```python
from build123d import *

# Parameters (mm, degrees)
ESBO_O1_R                = 10
RESSALTO_EXTRUS_O1_DEPTH = 6
RESSALTO_EXTRUS_O2_START = -4.5
RESSALTO_EXTRUS_O2_DEPTH = 4.5
FILETE1_R                = 3
FILETE2_R                = 1
FILETE3_R                = 10
ESBO_O3_R                = 4
RESSALTO_EXTRUS_O3_DEPTH = 10
ESBO_O4_R                = 3.3
CORTE_EXTRUS_O1_DEPTH    = 14


with BuildPart() as part:
    # Esboço1 → Ressalto-extrusão1 (new body)
    with BuildSketch(Plane.XY):
        Circle(ESBO_O1_R)
    extrude(amount=RESSALTO_EXTRUS_O1_DEPTH)

    # Esboço2 → Ressalto-extrusão2 (add)
    with BuildSketch(Plane.XY.offset(6).offset(RESSALTO_EXTRUS_O2_START)):
        with BuildLine():
            Line((-9.797958971, 2), (-37.5, 2))
            Line((-37.5, 2), (-37.5, -5))
            ThreePointArc((-37.5, -5), (-36, -6.5), (-34.5, -5))
            Line((-34.5, -5), (-34.5, -2))
            Line((-34.5, -2), (-9.797958971, -2))
            ThreePointArc((-9.797958971, -2), (-10, 0), (-9.797958971, 2))
        make_face()
    extrude(amount=RESSALTO_EXTRUS_O2_DEPTH)

    # Filete1
    filete1_edges = [part.edges().sort_by_distance(p)[0] for p in [
        (-37.5, 2, 3.75),
    ]]
    fillet(filete1_edges, radius=FILETE1_R)

    # Filete2
    filete2_edges = [part.edges().sort_by_distance(p)[0] for p in [
        (-34.5, -2, 3.75),
    ]]
    fillet(filete2_edges, radius=FILETE2_R)

    # Filete3
    filete3_edges = [part.edges().sort_by_distance(p)[0] for p in [
        (-9.797958971, 2, 3.75),
        (-9.797958971, -2, 3.75),
    ]]
    fillet(filete3_edges, radius=FILETE3_R)

    # Esboço3 → Ressalto-extrusão3 (add)
    with BuildSketch(Plane.XY.offset(6)):
        Circle(ESBO_O3_R)
    extrude(amount=RESSALTO_EXTRUS_O3_DEPTH)

    # Esboço4 → Corte-extrusão1 (cut)
    with BuildSketch(Plane.XY.offset(16)):
        Circle(ESBO_O4_R)
    extrude(amount=-CORTE_EXTRUS_O1_DEPTH, mode=Mode.SUBTRACT)


solid = part.part
```
Here's how the part is built. I have some questions about the finished solid (model axes, mm). A direction names the side the tool comes from. Coordinates: 2 decimals unless noted, no trailing zeros. Order: outer loops, then holes, each group sorted by start corner. A loop starts at its lowest first (then second) coordinate and runs counter-clockwise, first axis right, second up. Notation, with made-up numbers: (80, -5.75) -> (106, -5.75) arc R33 cw to (106, 27.25) -> close; hole circle Ø10 at (-23, 24). An arc over 180 degrees is marked (long way). Return JSON: item names as keys, results as strings.
1) If we section it at B-B on x = 0: List the corners of the cut face in (y, z) for me, plus the area to 3 significant figures.
Conclusion:
{"outline": "(-10, 0) -> (10, 0) -> (10, 6) -> (4, 6) -> (4, 16) -> (3.3, 16) -> (3.3, 2) -> (-3.3, 2) -> (-3.3, 16) -> (-4, 16) -> (-4, 6) -> (-10, 6) -> close", "area": "108 mm²"}
2) If we section it at A-A on z = 4.75: List the corners of the cut face in (x, y) for me.
Conclusion:
{"outline": "(-37.5, -5) arc R1.5 ccw to (-34.5, -5) -> (-34.5, -3) arc R1 cw to (-33.5, -2) -> (-16, -2) arc R10 cw to (-8, -6) arc R10 ccw (long way) to (-8, 6) arc R10 cw to (-16, 2) -> (-34.5, 2) arc R3 ccw to (-37.5, -1) -> close; hole circle Ø6.6 at (0, 0)"}
3) If I drill on probe 1 along Y at (x, z) = (0, 8); probe 2 along Z at (x, y) = (7.5, 6); probe 3 along Y at (x, z) = (8, 4), over which ranges is the centre line in solid material (lowest first)?
Conclusion:
{"probe 1": "y = -4 to -3.3, 3.3 to 4", "probe 2": "z = 0 to 6", "probe 3": "y = -6 to 6"}
4) Thinking about a two-plate mould opening in X: for faces 1 (the flat face through (-2, 3, 16)), 2 (the flat face through (0, 0, 2)), 3 (the cylindrical face through (-0.867, -3.905, 10.93)), which applies, +X half, -X half, draft (parallel to the pull), parting line (faces both ways), or undercut?
Conclusion:
{"face 1": "draft", "face 2": "undercut", "face 3": "parting line"}
5) I'm going to push flat-ended pins straight in: P1, Ø3.5, axis at x = -28, z = 4, coming from the +Y side; P2, Ø2, axis at x = -20.5, y = 1, coming from the +Z side; P3, Ø10, axis at x = -16, y = 1.5, coming from the -Z side. Where does each tip first touch, or does it pass through?
Conclusion:
{"P1": "stops at y = 2", "P2": "stops at z = 6", "P3": "stops at z = 1.5"}
6) If we section it at C-C on y = 0.5: List the corners of the cut face in (x, z) for me, plus the area to 3 significant figures.
Conclusion:
{"outline": "(-37.1, 1.5) -> (-9.99, 1.5) -> (-9.99, 0) -> (9.99, 0) -> (9.99, 6) -> (3.97, 6) -> (3.97, 16) -> (3.26, 16) -> (3.26, 2) -> (-3.26, 2) -> (-3.26, 16) -> (-3.97, 16) -> (-3.97, 6) -> (-37.1, 6) -> close", "area": "230 mm²"}
7) If we section it at D-D on z = 11: List the corners of the cut face in (x, y) for me, plus the area to 3 significant figures.
Conclusion:
{"outline": "circle Ø8 at (0, 0); hole circle Ø6.6 at (0, 0)", "area": "16.1 mm²"}
8) On a 3-axis mill with a long thin cutter (end or side, diameter ignored), from which of +Z, -Z, +X, -X, +Y, -Y can I reach the whole of each face in a straight line? I mean faces 4 (the cylindrical face through (-2.43, 2.23, 9.1)), 5 (the flat face through (-25, 2, 4)), 6 (the flat face through (-34.5, -4, 4)). Say none if no direction works.
Conclusion:
{"face 4": "+Z", "face 5": "+Z, -Z, -X, +Y", "face 6": "+Z, -Z, -Y"}
